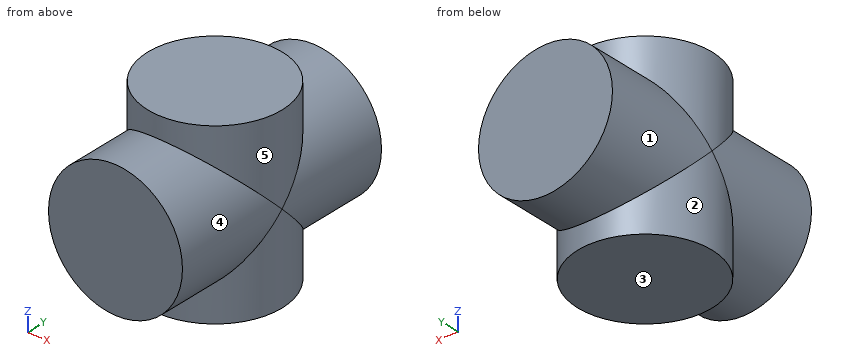
Solid Edge part; units mm, degrees
sketch "Sketch1" plane through (0, 0, 0) normal (0, -1, 0) x (1, 0, 0)
  circle A0 centre (0, 0) radius 8
extrude "Protrusion1" add sketch "Sketch1" against normal blind 28
sketch "Sketch2" plane through (0, 0, 0) normal (0, 0, -1) x (-1, 0, 0)
  circle A0 centre (0, 14) radius 8
extrude "ExtrudedProtrusion_2" add sketch "Sketch2" along normal blind 10.5
sketch "Sketch3" plane through (0, 0, 0) normal (0, 0, -1) x (-1, 0, 0)
  circle A0 centre (0, 14) radius 8
extrude "ExtrudedProtrusion_3" add sketch "Sketch3" against normal blind 10.5
Input: part model. Units: mm. Frame: model coordinates. Face numbers are marked on the shaded views. A direction names the side the tool comes from. Round coordinates to 2 decimals unless told otherwise and drop trailing zeros. Loops run counter-clockwise (first coordinate to the right, second up) from the corner with the lowest first, then second, coordinate; pieces in that order, holes last. Notation, with made-up numbers: (68.25, -23) -> (97.25, -23) arc R12 ccw to (97.25, -18) -> close; hole circle Ø1 at (-31.5, 83.5). An arc over 180 degrees is marked (long way). Answer as a JSON object with one key per item and string values. Group by question number.
1) Ray query, L1, parallel to X at y = 8.5, z = 1.5; L2, parallel to X at y = 24.75, z = -6; L3, parallel to Y at x = 5, z = -6.5 (3 decimals). Return the intervals inside material, ascending.
2) Section query A-A on x = 0. Output: boundary loops of the cut face in (y, z).
3) Pin query (flat end, axial travel): pin 1 (1 mm diameter, centred on x = -4, y = 4, fed in from -Z); pin 2 (1.5 mm diameter, centred on x = 0.5, z = 3, fed in from -Y); pin 3 (1.5 mm diameter, centred on x = -2.5, y = 5.5, fed in from -Z); pin 4 (5 mm diameter, centred on x = -1, y = 3.5, fed in from +Z). Return the tip coordinate at first contact, or that it passes through.
4) Section query B-B on z = -5.25. Output: boundary loops of the cut face in (x, y), plus the area to 3 significant figures.
5) Section query C-C on y = 7. Output: boundary loops of the cut face in (x, z), plus the area to 3 significant figures.
6) Section query D-D on x = 2.75. Output: boundary loops of the cut face in (y, z).
7) Reachability of the marked faces 1, 2, 3, 4 and 5 from +Z, -Z, +X, -X, +Y, -Y: full face, straight path, thin tool, end or side. Return the list, or none.
Reply:
{
 "1": {"L1": "x = -7.86 to 7.86", "L2": "x = -5.29 to 5.29", "L3": "y = 7.755 to 20.245"},
 "2": {"outline": "(0, -8) -> (6, -8) -> (6, -10.5) -> (22, -10.5) -> (22, -8) -> (28, -8) -> (28, 8) -> (22, 8) -> (22, 10.5) -> (6, 10.5) -> (6, 8) -> (0, 8) -> close"},
 "3": {"pin 1": "stops at z = -7.19", "pin 2": "stops at y = 0", "pin 3": "stops at z = -7.81", "pin 4": "stops at z = 8"},
 "4": {"outline": "(-6.04, 0) -> (6.04, 0) -> (6.04, 8.75) arc R8 ccw to (6.04, 19.25) -> (6.04, 28) -> (-6.04, 28) -> (-6.04, 19.25) arc R8 ccw to (-6.04, 8.75) -> close", "area": "366 mm2"},
 "5": {"outline": "(-3.87, -10.5) -> (3.87, -10.5) -> (3.87, -7) arc R8 ccw to (3.87, 7) -> (3.87, 10.5) -> (-3.87, 10.5) -> (-3.87, 7) arc R8 ccw to (-3.87, -7) -> close", "area": "245 mm2"},
 "6": {"outline": "(0, -7.51) -> (6.49, -7.51) -> (6.49, -10.5) -> (21.51, -10.5) -> (21.51, -7.51) -> (28, -7.51) -> (28, 7.51) -> (21.51, 7.51) -> (21.51, 10.5) -> (6.49, 10.5) -> (6.49, 7.51) -> (0, 7.51) -> close"},
 "7": {"face 1": "+Y", "face 2": "-Z", "face 3": "-Z, +X, -X, +Y, -Y", "face 4": "-Y", "face 5": "+Z"}
}
